from build123d import *

# Parameters (mm, degrees)
F0_R     = 3.45
F1_DEPTH = 81
F2_R     = 2.5
F3_DEPTH = 4.5
F0_R_2   = 4.5
F4_DEPTH = 1.9
F5_R     = 2.5
F6_DEPTH = 4.5
F7_SIZE  = 0.5


with BuildPart() as f1:
    # F0 (on Top) → F1 (new body)
    with BuildSketch(Plane.XY):
        Circle(F0_R)
    extrude(amount=F1_DEPTH)

    # F2 (on face) → F3 (join)
    with BuildSketch(Plane.XY.offset(81)):
        Circle(F2_R)
    extrude(amount=F3_DEPTH)

    # F0 (on Top) → F4 (join)
    with BuildSketch(Plane.XY):
        Circle(F0_R_2)
        Circle(F0_R, mode=Mode.SUBTRACT)
        Circle(F0_R)
    extrude(amount=-F4_DEPTH)

    # F5 (on face) → F6 (join)
    with BuildSketch(Plane(origin=(0, 0, -1.9), x_dir=(1, 0, 0), z_dir=(0, 0, -1))):
        Circle(F5_R)
    extrude(amount=F6_DEPTH)

    # F7
    f7_edges = [f1.edges().sort_by_distance(p)[0] for p in [
        (-2.5, 0, 85.5),
        (-3.45, 0, 81),
        (-2.5, 0, -6.4),
    ]]
    chamfer(f7_edges, length=F7_SIZE)


solid = f1.part
Build history of the part. All positions in model axes, mm. A direction names the side the tool comes from. Round coordinates to 2 decimals unless told otherwise and drop trailing zeros. Loops run counter-clockwise (first coordinate to the right, second up) from the corner with the lowest first, then second, coordinate; pieces in that order, holes last. Notation, with made-up numbers: (89, 37) -> (128, 37) arc R16 ccw to (128, 58) -> close; hole circle Ø6 at (31.25, -8). An arc over 180 degrees is marked (long way). One line per item, written item: value. Start each with the question number.
Q1. Drop flat-ended pins along their axis: pin 1 Ø4.5 at (x, y) = (2, 1.5) entering from -Z; pin 2 Ø5 at (x, z) = (-3, 41) entering from -Y; pin 3 Ø1.5 at (y, z) = (0.5, 61.5) entering from +X; pin 4 Ø5 at (x, y) = (3.5, -3.5) entering from +Z. Give the stop position or say it passes through.
Q2. Cut at A-A on y = 0. List the corners of the cut face in (x, z).
Q3. Cut at C-C on z = 54. List the corners of the cut face in (x, y).
Q4. 3-axis set-ups, long thin cutter, end or side, ignore diameter. For faces 1 (the face through (-0.54, -2.44, 82.97)), 2 (the face through (-0.59, 4.46, -0.94)), 3 (the face through (-0.54, 2.44, -3.87)): which of +Z, -Z, +X, -X, +Y, -Y reach the whole face in a straight line?
Q5. Probe line 1 along Z through (x, y) = (-1, -3.5); line 2 along Z through (x, y) = (2.5, 0.5); line 3 along X through (y, z) = (1, 18.5). List the from-to ranges inside material, lowest first.
Computed:
1. pin 1: z = -6.4
1. pin 2: y = -3.41
1. pin 3: x = 3.45
1. pin 4: z = 85.05
2. outline: (-4.5, -1.9) -> (-2.5, -1.9) -> (-2.5, -5.9) -> (-2, -6.4) -> (2, -6.4) -> (2.5, -5.9) -> (2.5, -1.9) -> (4.5, -1.9) -> (4.5, 0) -> (3.45, 0) -> (3.45, 80.5) -> (2.95, 81) -> (2.5, 81) -> (2.5, 85) -> (2, 85.5) -> (-2, 85.5) -> (-2.5, 85) -> (-2.5, 81) -> (-2.95, 81) -> (-3.45, 80.5) -> (-3.45, 0) -> (-4.5, 0) -> close
3. outline: circle Ø6.9 at (0, 0)
4. face 1: +Z
4. face 2: +Z, -Z
4. face 3: -Z
5. line 1: -1.9 to 0
5. line 2: -1.9 to 81
5. line 3: -3.3 to 3.3
